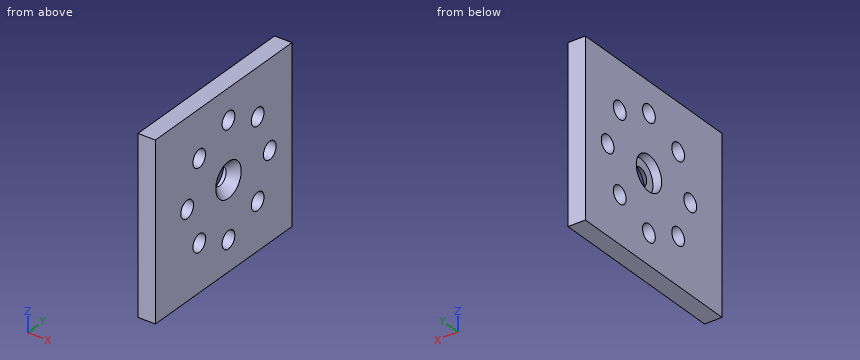
from build123d import *

# Parameters (mm, degrees)
ESQUISSE1_W      = 4
ESQUISSE1_H      = 43
EXTRUSION1_DEPTH = 40
ESQUISSE2_R      = 2
EXTRUSION2_DEPTH = 59.864250611
ESQUISSE3_R      = 4
EXTRUSION3_DEPTH = 2
CHANFREIN1_SIZE  = 2


with BuildPart() as part:
    # Esquisse1 → Extrusion1 (new body)
    with BuildSketch(Plane.XY):
        with Locations((2, 21.5)):
            Rectangle(ESQUISSE1_W, ESQUISSE1_H)
    extrude(amount=EXTRUSION1_DEPTH)

    # Esquisse2 → Extrusion2 (cut, through all)
    with BuildSketch(Plane.ZY):
        with Locations((29.192388155, 32.192388155)):
            Circle(ESQUISSE2_R)
        with Locations((20, 23)):
            Circle(ESQUISSE2_R)
        with Locations((20, 36)):
            Circle(ESQUISSE2_R)
        with Locations((33, 23)):
            Circle(ESQUISSE2_R)
        with Locations((29.192388155, 13.807611845)):
            Circle(ESQUISSE2_R)
        with Locations((20, 10)):
            Circle(ESQUISSE2_R)
        with Locations((10.807611845, 13.807611845)):
            Circle(ESQUISSE2_R)
        with Locations((7, 23)):
            Circle(ESQUISSE2_R)
        with Locations((10.807611845, 32.192388155)):
            Circle(ESQUISSE2_R)
    extrude(amount=-EXTRUSION2_DEPTH, mode=Mode.SUBTRACT)

    # Esquisse3 → Extrusion3 (cut)
    with BuildSketch(Plane.ZY):
        with Locations((20, 23)):
            Circle(ESQUISSE3_R)
    extrude(amount=-EXTRUSION3_DEPTH, mode=Mode.SUBTRACT)

    # Chanfrein1
    chanfrein1_edges = [part.edges().sort_by_distance(p)[0] for p in [
        (4, 23, 18),
    ]]
    chamfer(chanfrein1_edges, length=CHANFREIN1_SIZE - 0.0001)  # a hair under: the kernel refuses the full size


solid = part.part
Geometry: final body of the model. Coordinates: model frame, mm. Coordinates: 2 decimals unless noted, no trailing zeros. Loops run counter-clockwise (first coordinate to the right, second up) from the corner with the lowest first, then second, coordinate; pieces in that order, holes last. Notation, with made-up numbers: M 37,-8 L 52,-8 A25 cw 52,18 Z; hole C 32.5,20 d2. An arc over 180 degrees is marked long. One line per item, written item: value. Start each with the question number.
1) Cut plane B-B (z = 20). Count the separate pieces of the cut face and the enclosed holes in it, then the cut area to 3 significant figures.
2) Pin query (flat end, axial travel): P1, Ø6.5, axis at y = 23, z = 20, coming from the +X side; P2, Ø1.5, axis at y = 21.5, z = 28, coming from the -X side; P3, Ø2.5, axis at y = 22, z = 22, coming from the -X side. Return the tip coordinate at first contact, or that it passes through.
3) Material intervals for L1, parallel to Z at x = 1.3, y = 32.5; L2, parallel to Y at x = 3.75, z = 10.5; L3, parallel to Y at x = 2.8, z = 7, sorted ascending. Write a range as from..to.
4) Cut plane D-D (y = 36). Return loops of the section in (x, z).
5) Cut plane A-A (z = 7). Return loops of the section in (x, y).
Evaluation:
1. separate pieces: 4
1. enclosed holes: 0
1. area: 112 mm^2
2. P1: x = 3.25
2. P2: x = 0
2. P3: x = 2
3. L1: 0..8.83, 12.78..27.22, 31.17..40
3. L2: 0..11.83, 15.78..30.22, 34.17..43
3. L3: 0..21, 25..43
4. outline: M 0,0 L 4,0 L 4,18 L 0,18 Z; M 0,22 L 4,22 L 4,40 L 0,40 Z
5. outline: M 0,0 L 4,0 L 4,21 L 0,21 Z; M 0,25 L 4,25 L 4,43 L 0,43 Z
